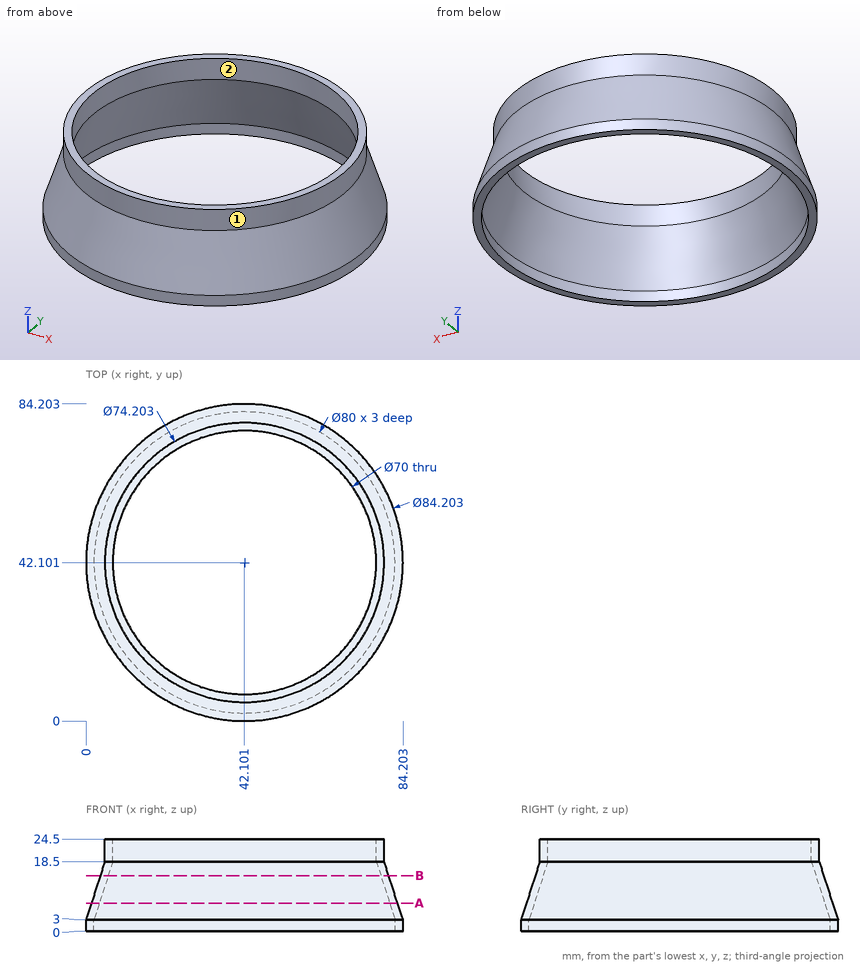
Check sheet for the drawn part. Datum: minimum x, y, z corner. Units: mm. A direction names the side the tool comes from. Coordinates: 2 decimals unless noted, no trailing zeros. Loops run counter-clockwise (first coordinate to the right, second up) from the corner with the lowest first, then second, coordinate; pieces in that order, holes last. Notation, with made-up numbers: (5.25, -23.75) -> (39.25, -23.75) arc R32 ccw to (39.25, 15.25) -> close; hole circle Ø11 at (-32, -29). An arc over 180 degrees is marked (long way). Answer as CSV lines item,"result".
1) Depth check by flat-ended pin: pin 1 (12 mm diameter, centred on y = 71, z = 3, fed in from -X); pin 2 (3 mm diameter, centred on y = 10, z = 11, fed in from -X); pin 3 (6 mm diameter, centred on x = 51, z = 17, fed in from +Y) (1 decimal). Enter the tip coordinate at first touch or a pass-through.
Found:
pin 1,"stops at x = 6.77"
pin 2,"stops at x = 16.94"
pin 3,"stops at y = 79.8"
2) Tool access check on the marked faces 1 and 2. Record the directions out of +Z, -Z, +X, -X, +Y, -Y that give a thin tool (end or side, any length) a straight path to the whole face; none if there is none.
Found:
face 1,"+Z"
face 2,"+Z, -Z"
3) Cross-section at B-B, the plane z = 14.75. Record the cut outline in (x, y).
Found:
outline,"circle Ø76.62 at (42.1, 42.1); hole circle Ø72.42 at (42.1, 42.1)"
4) Thickness scan on L1, parallel to X at y = 67.5, z = 21.25 (1 decimal); L2, parallel to Y at x = 53, z = 7.75 (1 decimal); L3, parallel to X at y = 16, z = 22.5 (1 decimal). Record the ranges inside material, lowest first. Write a range as from..to.
Found:
L1,"x = 15.1..18, 66.2..69.1"
L2,"y = 3..5.2, 79..81.2"
L3,"x = 15.7..18.8, 65.4..68.5"
5) Cross-section at A-A, the plane z = 7.5. Record the cut outline in (x, y).
Found:
outline,"circle Ø81.3 at (42.1, 42.1); hole circle Ø77.1 at (42.1, 42.1)"
